```python
from build123d import *

# Parameters (mm, degrees)
F0_W     = 300
F0_H     = 110
F1_DEPTH = 25
F2_R     = 5
F3_DEPTH = 25.001
F4_R     = 5


with BuildPart() as f1:
    # F0 (on Top) → F1 (new body)
    with BuildSketch(Plane.XY):
        Rectangle(F0_W, F0_H)
    extrude(amount=F1_DEPTH)

    # F2 (on face) → F3 (cut, through all)
    with BuildSketch(Plane.XY.offset(25)):
        with Locations((-112.5, 35)):
            Circle(F2_R)
        with Locations((-112.5, -35)):
            Circle(F2_R)
        with Locations((112.5, -35)):
            Circle(F2_R)
        with Locations((112.5, 35)):
            Circle(F2_R)
    extrude(amount=-F3_DEPTH, mode=Mode.SUBTRACT)

    # F4
    f4_edges = [f1.edges().sort_by_distance(p)[0] for p in [
        (0, 55, 25),
        (-150, 0, 25),
        (0, -55, 25),
        (150, 0, 25),
        (150, 0, 0),
        (0, 55, 0),
        (-150, 0, 0),
        (-150, -55, 12.5),
        (-150, 55, 12.5),
        (150, 55, 12.5),
        (150, -55, 12.5),
        (0, -55, 0),
    ]]
    fillet(f4_edges, radius=F4_R)


solid = f1.part
```
Work out the finished part from the listing and answer in its coordinate system (mm). Give positions to 0.01 mm unless a question says otherwise; leave off trailing zeros. Write each loop counter-clockwise with the first axis right and the second up, starting at its lowest first coordinate (ties: lowest second). Pieces come first, ordered by that corner, then holes. Notation, with made-up numbers: (-25, 14) -> (22, 14) arc R26 ccw to (22, 45) -> close; hole circle Ø5 at (-38.5, -2). An arc over 180 degrees is marked (long way). Write each question's results on one line, items separated by ' | '.
1. Straight lines are drawn through the part: L1, parallel to Y at x = 112.5, z = 8.25; L2, parallel to X at y = -32.5, z = 18.25; L3, parallel to X at y = 39, z = 17. For each, find the intervals that lie inside material, in ascending order.
Data:
L1: -55 to -40, -30 to 30, 40 to 55 | L2: -150 to -116.83, -108.17 to 108.17, 116.83 to 150 | L3: -150 to -115.5, -109.5 to 109.5, 115.5 to 150
2. This flat-tipped pin is pushed along its axis until it touches: pin 1 Ø8 at (x, y) = (-112.5, -35) entering from -Z. Where does it stop, or does it pass through?
Data:
pin 1: through
3. Determine the mould class of faces 1 (the cylindrical face through (-149, -53, 13)), 2 (the flat face through (150, -1, 12)), 3 (the cylindrical face through (-107.73, 36.5, 12.68)) for opening direction Y: +Y half, -Y half, draft (parallel to the pull), parting line (faces both ways), or undercut.
Data:
face 1: -Y half | face 2: draft | face 3: undercut
4. Find section A-A on x = -112.5. Determine the outline of the cut face in (y, z).
Data:
outline: (-55, 5) arc R5 ccw to (-50, 0) -> (-40, 0) -> (-40, 25) -> (-50, 25) arc R5 ccw to (-55, 20) -> close; (-30, 0) -> (30, 0) -> (30, 25) -> (-30, 25) -> close; (40, 0) -> (50, 0) arc R5 ccw to (55, 5) -> (55, 20) arc R5 ccw to (50, 25) -> (40, 25) -> close
5. Find section B-B on y = -35. Determine the outline of the cut face in (x, z).
Data:
outline: (-150, 5) arc R5 ccw to (-145, 0) -> (-117.5, 0) -> (-117.5, 25) -> (-145, 25) arc R5 ccw to (-150, 20) -> close; (-107.5, 0) -> (107.5, 0) -> (107.5, 25) -> (-107.5, 25) -> close; (117.5, 0) -> (145, 0) arc R5 ccw to (150, 5) -> (150, 20) arc R5 ccw to (145, 25) -> (117.5, 25) -> close
